Source: CAD feature listing. Evaluate the final solid. Frame: model axes, mm. Give positions to 0.01 mm unless a question says otherwise; leave off trailing zeros. Loops run counter-clockwise (first coordinate to the right, second up) from the corner with the lowest first, then second, coordinate; pieces in that order, holes last. Notation, with made-up numbers: M 33,-24.5 L 90,-24.5 A30 ccw 90,3.5 Z; hole C 50,40.5 d3. An arc over 180 degrees is marked long. Put each result on its own line as item: value.
from build123d import *


# Read off the part's stored shape, not the designer's step: Shell2
with BuildPart() as part:
    # Sketch1 → Revolve1 (revolve)
    with BuildSketch(Plane.XY, mode=Mode.PRIVATE) as revolve1_sk:
        with BuildLine():
            Line((-6.6675, 0), (-6.6675, 0.635))
            Line((-6.6675, 0.635), (-5.5245, 0.635))
            Line((-5.5245, 0.635), (-5.086993169, 2.438135229))
            ThreePointArc((-5.086993169, 2.438135229), (-4.740640087, 2.78173227), (-4.277735634, 2.627658097))
            Line((-4.277735634, 2.627658097), (-2.286, 0.254))
            Line((-2.286, 0.254), (-2.286, 0))
            Line((-2.286, 0), (-6.6675, 0))
        make_face()
    revolve(revolve1_sk.sketch.rotate(Axis((0, 0, 0), (0, 1, 0)), 270), axis=Axis((0, 0, 0), (0, 1, 0)))

    # Shell2 outline → Shell2 (revolve, cut)
    with BuildSketch(Plane.XY):
        Polygon((4.861793391, 0), (4.468644562, 1.620318711), (3.10903573, 0), align=None)
    revolve(axis=Axis((0, 0, 0), (0, 1, 0)), mode=Mode.SUBTRACT)


solid = part.part
1. Section query C-C (y = 1.45). Output: boundary loops of the cut face in (x, z), plus the area to 3 significant figures.
Found:
outline: C 0,0 d10.65; C 0,0 d8.65; hole C 0,0 d9.02; hole C 0,0 d6.58
area: 50.0 mm^2
2. Draft query along Z for faces 1 (the cylindrical face through (-6.61, 0.32, 0.87)), 2 (the flat face through (-5, 0.635, 3)), 3 (the conical face through (-0.72, 0.37, -2.27)). Return one class per face: pulls with the +Z half, pulls with the -Z half, needs draft (parallel to the pull), parting line crosses it, or undercut.
Found:
face 1: parting line crosses it
face 2: needs draft
face 3: undercut
3. Contact query for flat-ended pins moving along their axis: P1, Ø1, axis at y = 2.5, z = 0, coming from the +X side; P2, Ø4, axis at x = -0.5, z = 0.5, coming from the +Y side. Output: stop coordinate, or through.
Found:
P1: x = 5.19
P2: y = 0.76
4. Material intervals for line 1 (X direction, y = 0.5, z = -3); line 2 (X direction, y = 0.1, z = 0); line 3 (Y direction, x = -1.5, z = 5.5) (3 decimals), sorted ascending. Write a range as from..to.
Found:
line 1: -5.95..-3.67, -1.86..1.86, 3.67..5.95
line 2: -6.67..-4.84, -3.19..-2.29, 2.29..3.19, 4.84..6.67
line 3: 0..0.635
